The model under review builds one solid part; all positions refer to its coordinate system, in mm. A direction names the side the tool comes from. Round coordinates to 2 decimals unless told otherwise and drop trailing zeros. Order: outer loops, then holes, each group sorted by start corner. A loop starts at its lowest first (then second) coordinate and runs counter-clockwise, first axis right, second up.
```python
from build123d import *

# Parameters (mm, degrees)
SKETCH1_R      = 4.25
SKETCH1_R_2    = 1.75
SKETCH1_W      = 8.5
SKETCH1_H      = 8.5
EXTRUDE1_DEPTH = 8
SKETCH2_R      = 1.75
EXTRUDE2_DEPTH = 10


with BuildPart() as part:
    # Sketch1 → Extrude1 (new body)
    with BuildSketch(Plane.XY):
        with BuildLine():
            Line((5.082943524, 52.898094917), (5.082943524, 10.898094917))
            ThreePointArc((5.082943524, 10.898094917), (6.840302837, 6.65545423), (11.082943524, 4.898094917))
            Line((11.082943524, 4.898094917), (40.082943524, 4.898094917))
            Line((40.082943524, 4.898094917), (43.082943524, 7.898094917))
            Line((43.082943524, 7.898094917), (161.082943524, 7.898094917))
            Line((161.082943524, 7.898094917), (164.082943524, 4.898094917))
            Line((164.082943524, 4.898094917), (193.082943524, 4.898094917))
            ThreePointArc((193.082943524, 4.898094917), (197.325584211, 6.65545423), (199.082943524, 10.898094917))
            Line((199.082943524, 10.898094917), (199.082943524, 52.898094917))
            ThreePointArc((199.082943524, 52.898094917), (197.325584211, 57.140735604), (193.082943524, 58.898094917))
            Line((193.082943524, 58.898094917), (11.082943524, 58.898094917))
            ThreePointArc((11.082943524, 58.898094917), (6.840302837, 57.140735604), (5.082943524, 52.898094917))
        make_face()
        with Locations((186.582943524, 50.398094917)):
            Circle(SKETCH1_R, mode=Mode.SUBTRACT)
        with Locations((186.582943524, 24.398094917)):
            Circle(SKETCH1_R, mode=Mode.SUBTRACT)
        with Locations((17.582943524, 50.398094917)):
            Circle(SKETCH1_R, mode=Mode.SUBTRACT)
        with Locations((17.582943524, 24.398094917)):
            Circle(SKETCH1_R, mode=Mode.SUBTRACT)
        with Locations((92.832943524, 31.898094917)):
            Circle(SKETCH1_R_2, mode=Mode.SUBTRACT)
        with Locations((111.332943524, 31.898094917)):
            Circle(SKETCH1_R_2, mode=Mode.SUBTRACT)
        with Locations((92.832943524, 40.648094917)):
            Rectangle(SKETCH1_W, SKETCH1_H, mode=Mode.SUBTRACT)
        with Locations((111.332943524, 40.648094917)):
            Rectangle(SKETCH1_W, SKETCH1_H, mode=Mode.SUBTRACT)
        with Locations((92.832943524, 23.148094917)):
            Rectangle(SKETCH1_W, SKETCH1_H, mode=Mode.SUBTRACT)
        with Locations((111.332943524, 23.148094917)):
            Rectangle(SKETCH1_W, SKETCH1_H, mode=Mode.SUBTRACT)
    extrude(amount=EXTRUDE1_DEPTH)

    # Sketch2 → Extrude2 (cut)
    with BuildSketch(Plane.XY.offset(8)):
        with Locations((28.189545242, 39.791493199)):
            Circle(SKETCH2_R)
        with Locations((175.976341806, 39.791493199)):
            Circle(SKETCH2_R)
    extrude(amount=-EXTRUDE2_DEPTH, mode=Mode.SUBTRACT)


solid = part.part
```
(1) Insertion check: pin 1 (4 mm diameter, centred on x = 94, z = 4, fed in from -Y). The pin has a flat end and moves straight along its axis. Give the tip position at first contact, or say it passes through.
Data:
pin 1: stops at y = 7.9
(2) Consider section C-C (z = 5.5). State how many separate pieces and enclosed holes the cut face has, and give its area (3 significant figures).
Data:
separate pieces: 1
enclosed holes: 12
area: 9,530 mm2
(3) For faces 1 (the flat face through (93, 44.898, 4)), 2 (the flat face through (103, 58.898, 4)), list the 3-axis set-ups (+Z, -Z, +X, -X, +Y, -Y) from which the entire face can be reached by the end or side of a thin tool; tool diameter is ignored.
Data:
face 1: +Z, -Z
face 2: +Z, -Z, +X, -X, +Y
(4) Draft analysis for pull direction Y (two halves, no side actions). For faces 3 (the flat face through (101, 7.898, 4)), 4 (the flat face through (101, 32, 0)), 5 (the flat face through (93, 18.898, 4)), 6 (the flat face through (107.083, 23, 4)), state which applies: pulls with the +Y half, pulls with the -Y half, needs draft (parallel to the pull), parting line crosses it, or undercut.
Data:
face 3: pulls with the -Y half
face 4: needs draft
face 5: undercut
face 6: undercut
(5) Consider section A-A (y = 22.5). Write out the cut boundary in (x, z), and give its area (3 significant figures).
Data:
outline: (5.08, 0) - (13.78, 0) - (13.78, 8) - (5.08, 8) - close; (21.39, 0) - (88.58, 0) - (88.58, 8) - (21.39, 8) - close; (97.08, 0) - (107.08, 0) - (107.08, 8) - (97.08, 8) - close; (115.58, 0) - (182.78, 0) - (182.78, 8) - (115.58, 8) - close; (190.39, 0) - (199.08, 0) - (199.08, 8) - (190.39, 8) - close
area: 1,290 mm2
(6) To check wall thickness, follow probe 1 along X at (y, z) = (50.5, 3.25); probe 2 along X at (y, z) = (40, 1.75); probe 3 along X at (y, z) = (22.5, 2.75). State the ranges of each line that lie inside material, in increasing order.
Data:
probe 1: x = 5.08 to 13.33, 21.83 to 182.33, 190.83 to 199.08
probe 2: x = 5.08 to 26.45, 29.93 to 88.58, 97.08 to 107.08, 115.58 to 174.24, 177.71 to 199.08
probe 3: x = 5.08 to 13.78, 21.39 to 88.58, 97.08 to 107.08, 115.58 to 182.78, 190.39 to 199.08
(7) Consider section B-B (x = 147.5). Write out the cut boundary in (y, z), and give its area (3 significant figures).
Data:
outline: (7.9, 0) - (58.9, 0) - (58.9, 8) - (7.9, 8) - close
area: 408 mm2
